from build123d import *

# Parameters (mm, degrees)
SKETCH1_W               = 20
SKETCH1_H               = 300
BOSS_EXTRUDE1_DEPTH     = 3.175
SKETCH2_R               = 2
SKETCH2_R_2             = 2.032
BOSS_EXTRUDE2_DEPTH     = 3.175
SKETCH4_R               = 2
CUT_EXTRUDE1_DEPTH      = 153.248468794
SKETCH6_R               = 2.032
BOSS_EXTRUDE4_DEPTH     = 3.175
FILLET4_R               = 0.79375
SKETCH7_R               = 4.7625
SKETCH7_R_2             = 6.985
SKETCH7_R_3             = 2.032
BOSS_EXTRUDE5_DEPTH     = 3.175
SKETCH8_R               = 2.032
CUT_EXTRUDE2_DEPTH      = 164.103897102
CUT_EXTRUDE3_DEPTH      = 164.103897102
SKETCH10_R              = 2.032
CUT_EXTRUDE4_DEPTH      = 164.103897102
FILLET6_R               = 6.35
CUT_EXTRUDE5_DEPTH      = 164.103897102
CUT_EXTRUDE5_DEPTH_BACK = 164.103897102
SKETCH11_R              = 2
SKETCH12_R              = 2.032
BOSS_EXTRUDE6_DEPTH     = 3.175
FILLET7_R               = 0.79375


with BuildPart() as part:
    # Sketch1 → Boss-Extrude1 (new body)
    with BuildSketch(Plane.XY):
        Rectangle(SKETCH1_W, SKETCH1_H)
    extrude(amount=BOSS_EXTRUDE1_DEPTH)

    # Sketch2 → Boss-Extrude2 (add)
    # profile 1 of 2: a face of its own
    with BuildSketch(Plane.XY.offset(3.175)):
        Polygon((10, 150), (25.875, 143.65), (25.875, 124.6), (10, 118.25), align=None)
        with Locations((17.9375, 140.475)):
            Circle(SKETCH2_R, mode=Mode.SUBTRACT)
        with Locations((17.9375, 127.775)):
            Circle(SKETCH2_R_2, mode=Mode.SUBTRACT)
    # profile 2 of 2: a face of its own
    with BuildSketch(Plane.XY.offset(3.175)):
        Polygon((10, -118.25), (10, -150), (25.875, -143.65), (25.875, -124.6), align=None)
        with Locations((17.9375, -127.775)):
            Circle(SKETCH2_R, mode=Mode.SUBTRACT)
        with Locations((17.9375, -140.475)):
            Circle(SKETCH2_R, mode=Mode.SUBTRACT)
    extrude(amount=-BOSS_EXTRUDE2_DEPTH)

    # Sketch4 → Cut-Extrude1 (cut, through all)
    with BuildSketch(Plane.XY.offset(3.175)):
        with Locations((0, -135)):
            Circle(SKETCH4_R)
        Circle(SKETCH4_R)
        with Locations((0, 135)):
            Circle(SKETCH4_R)
    extrude(amount=-CUT_EXTRUDE1_DEPTH, mode=Mode.SUBTRACT)

    # Sketch6 → Boss-Extrude4 (add)
    with BuildSketch(Plane.XY.offset(3.175)):
        with BuildLine():
            Line((-10, -124.6), (-10, -150))
            Line((-10, -150), (-25.875, -150))
            ThreePointArc((-25.875, -150), (-33.575506095, -143.987626524), (-29.610294118, -135.058823529))
            Line((-29.610294118, -135.058823529), (-10, -124.6))
        make_face()
        with Locations((-25.875, -142.0625)):
            Circle(SKETCH6_R, mode=Mode.SUBTRACT)
    extrude(amount=-BOSS_EXTRUDE4_DEPTH)

    # Fillet4
    fillet4_edges = [part.edges().sort_by_distance(p)[0] for p in [
        (25.875, 124.6, 1.5875),
        (25.875, 143.65, 1.5875),
        (10, 118.25, 1.5875),
        (25.875, -143.65, 1.5875),
        (25.875, -124.6, 1.5875),
        (10, -118.25, 1.5875),
        (-10, -124.6, 1.5875),
        (-10, 150, 1.5875),
    ]]
    fillet(fillet4_edges, radius=FILLET4_R)

    # Sketch7 → Boss-Extrude5 (add)
    with BuildSketch(Plane(origin=(0, 0, 0), x_dir=(-1, 0, 0), z_dir=(0, 0, -1))):
        with BuildLine():
            Line((-25.533906668, 143.764633463), (-63.633906668, 117.314528376))
            ThreePointArc((-63.633906668, 117.314528376), (-63.884576131, 117.030428547), (-63.975, 116.6625))
            Line((-63.975, 116.6625), (-63.975, 10.1095))
            ThreePointArc((-63.975, 10.1095), (-63.318896855, 8.176682463), (-61.621750468, 7.042685502))
            Line((-61.621750468, 7.042685502), (-10, -6.789320848))
            Line((-10, -6.789320848), (-10, 117.712605087))
            ThreePointArc((-10, 117.712605087), (-10.136471636, 118.157604204), (-10.498958651, 118.44958346))
            Line((-10.498958651, 118.44958346), (-25.376041349, 124.40041654))
            ThreePointArc((-25.376041349, 124.40041654), (-25.738528364, 124.692395796), (-25.875, 125.137394913))
            Line((-25.875, 125.137394913), (-25.875, 143.112605087))
            ThreePointArc((-25.875, 143.112605087), (-25.784576131, 143.480533634), (-25.533906668, 143.764633463))
        make_face()
        with Locations((-47.4015, 99.2)):
            Circle(SKETCH7_R, mode=Mode.SUBTRACT)
        with Locations((-47.4015, 48.4)):
            Circle(SKETCH7_R_2, mode=Mode.SUBTRACT)
        with Locations((-57.72025, 67.45)):
            Circle(SKETCH7_R_3, mode=Mode.SUBTRACT)
        with Locations((-57.72025, 23)):
            Circle(SKETCH7_R_3, mode=Mode.SUBTRACT)
        with Locations((-37.08275, 23)):
            Circle(SKETCH7_R_3, mode=Mode.SUBTRACT)
        with Locations((-37.08275, 67.45)):
            Circle(SKETCH7_R_3, mode=Mode.SUBTRACT)
        with Locations((-18.73125, 10.3)):
            Circle(SKETCH7_R_3, mode=Mode.SUBTRACT)
    extrude(amount=-BOSS_EXTRUDE5_DEPTH)

    # Sketch8 → Cut-Extrude2 (cut, through all)
    with BuildSketch(Plane.XY.offset(3.175)):
        with Locations((47.4015, 67.45)):
            Circle(SKETCH8_R)
        with Locations((28.3515, 48.4)):
            Circle(SKETCH8_R)
        with Locations((47.4015, 29.35)):
            Circle(SKETCH8_R)
        with Locations((56.9265, 99.2)):
            Circle(SKETCH8_R)
        with Locations((37.8765, 99.2)):
            Circle(SKETCH8_R)
        with Locations((18.03275, 54.75)):
            Circle(SKETCH8_R)
        with Locations((18.03275, 67.45)):
            Circle(SKETCH8_R)
    extrude(amount=-CUT_EXTRUDE2_DEPTH, mode=Mode.SUBTRACT)

    # Sketch9 → Cut-Extrude3 (cut, through all)
    with BuildSketch(Plane(origin=(0, 0, 0), x_dir=(-1, 0, 0), z_dir=(0, 0, -1))):
        with BuildLine():
            Line((-25.644749354, 143.671628825), (-58.67148709, 110.380474766))
            ThreePointArc((-58.67148709, 110.380474766), (-61.914239932, 105.633972698), (-63.254057026, 100.043836919))
            Line((-63.254057026, 100.043836919), (-63.975, 86.5))
            Line((-63.975, 86.5), (-63.975, 116.6625))
            ThreePointArc((-63.975, 116.6625), (-63.884576131, 117.030428547), (-63.633906668, 117.314528376))
            Line((-63.633906668, 117.314528376), (-25.533906668, 143.764633463))
            ThreePointArc((-25.533906668, 143.764633463), (-25.591451658, 143.7206621), (-25.644749354, 143.671628825))
        make_face()
    extrude(amount=-CUT_EXTRUDE3_DEPTH, mode=Mode.SUBTRACT)

    # Sketch10 → Cut-Extrude4 (cut, through all)
    with BuildSketch(Plane(origin=(0, 0, 0), x_dir=(-1, 0, 0), z_dir=(0, 0, -1))):
        with Locations((-57.625, 84.9125)):
            Circle(SKETCH10_R)
        with Locations((-44.925, 84.9125)):
            Circle(SKETCH10_R)
    extrude(amount=-CUT_EXTRUDE4_DEPTH, mode=Mode.SUBTRACT)

    # Fillet6
    fillet6_edges = [part.edges().sort_by_distance(p)[0] for p in [
        (10, -6.789320848, 1.5875),
    ]]
    fillet(fillet6_edges, radius=FILLET6_R)

    # Sketch11 → Cut-Extrude5 (cut, two sides: drawn at the far end of the back side and taken through both)
    with BuildSketch(Plane.XY.offset(3.175).offset(-CUT_EXTRUDE5_DEPTH_BACK)):
        with BuildLine():
            ThreePointArc((10.498958651, -118.44958346), (10.136471636, -118.157604204), (10, -117.712605087))
            Line((10, -117.712605087), (10, -150))
            Line((10, -150), (25.376041349, -143.84958346))
            ThreePointArc((25.376041349, -143.84958346), (25.738528364, -143.557604204), (25.875, -143.112605087))
            Line((25.875, -143.112605087), (25.875, -125.137394913))
            ThreePointArc((25.875, -125.137394913), (25.738528364, -124.692395796), (25.376041349, -124.40041654))
            Line((25.376041349, -124.40041654), (10.498958651, -118.44958346))
        make_face()
        with Locations((17.9375, -140.475)):
            Circle(SKETCH11_R, mode=Mode.SUBTRACT)
        with Locations((17.9375, -127.775)):
            Circle(SKETCH11_R, mode=Mode.SUBTRACT)
    extrude(amount=CUT_EXTRUDE5_DEPTH + CUT_EXTRUDE5_DEPTH_BACK, mode=Mode.SUBTRACT)

    # Sketch12 → Boss-Extrude6 (add)
    with BuildSketch(Plane.XY.offset(3.175)):
        Polygon((10, -150), (25.875, -143.65), (25.875, -130.95), (10, -124.6), align=None)
        with Locations((17.9375, -137.3)):
            Circle(SKETCH12_R, mode=Mode.SUBTRACT)
    extrude(amount=-BOSS_EXTRUDE6_DEPTH)

    # Fillet7
    fillet7_edges = [part.edges().sort_by_distance(p)[0] for p in [
        (25.875, -143.65, 1.5875),
        (25.875, -130.95, 1.5875),
        (10, -124.6, 1.5875),
        (10, -150, 1.5875),
    ]]
    fillet(fillet7_edges, radius=FILLET7_R)


solid = part.part
For this review, take the finished solid that the model builds, in its own axes (mm). A direction names the side the tool comes from. Round coordinates to 2 decimals unless told otherwise and drop trailing zeros. Loops run counter-clockwise (first coordinate to the right, second up) from the corner with the lowest first, then second, coordinate; pieces in that order, holes last. Notation, with made-up numbers: (-9.75, 29.5) - (17.25, 29.5) arc R20 cw to (17.25, 62.5) - close; hole circle Ø7 at (19, 79.5). An arc over 180 degrees is marked (long way). Use one line per item in the form item = value.
1) We need section A-A on y = -61.5. Write out the cut boundary in (x, z) (3 decimals).
Solutions:
outline = (-10, 0) - (10, 0) - (10, 3.175) - (-10, 3.175) - close
2) We need section B-B on z = 1.2. State how many separate pieces and enclosed holes the cut face has, then the cut area to 3 significant figures.
Solutions:
separate_pieces = 1
enclosed_holes = 23
area = 13,300 mm2
3) Wall thickness on probe 1 along Y at (x, z) = (49.5, 1.3); probe 2 along Y at (x, z) = (37, 1.15); probe 3 along Y at (x, z) = (24, 0.2): over which ranges is each line inside the solid? List them lowest first.
Solutions:
probe_1 = 3.79 to 41.74, 55.06 to 94.92, 103.48 to 119.63
probe_2 = 0.45 to 20.97, 25.03 to 65.42, 69.48 to 97.37, 101.03 to 132.23
probe_3 = -144.4 to -130.2, -3.04 to 144.4
4) Tool access review of faces 1 (the face through (18, -127.8, 1.6)), 2 (the face through (14, 2, 0)): name each direction out of +Z, -Z, +X, -X, +Y, -Y from which nothing blocks a thin tool from reaching the whole face with its end or side.
Solutions:
face_1 = +Z, -Z, +X
face_2 = -Z, +X, -X, +Y, -Y
5) Clearance check with flat-ended pins moving along their axes: P1, Ø1, axis at y = -136.5, z = 2.5, coming from the +X side (3 decimals); P2, Ø1.6, axis at y = 69.5, z = 2, coming from the -X side. State where each tip first meets the part, or that it passes through.
Solutions:
P1 = 25.875
P2 = -10
6) Mouldability with a two-part tool opening along Y and no side actions: class faces 3 (the face through (38.493, 0.845, 1.565)), 4 (the face through (41.927, 127.259, 1.565)), 5 (the face through (17.65, -146.94, 1.61)) as pulls with the +Y half, pulls with the -Y half, needs draft (parallel to the pull), parting line crosses it, or undercut.
Solutions:
face_3 = undercut
face_4 = pulls with the +Y half
face_5 = pulls with the -Y half
7) We need section C-C on x = -17. Write out the cut boundary in (y, z) (3 decimals).
Solutions:
outline = (-150, 0) - (-128.333, 0) - (-128.333, 3.175) - (-150, 3.175) - close
